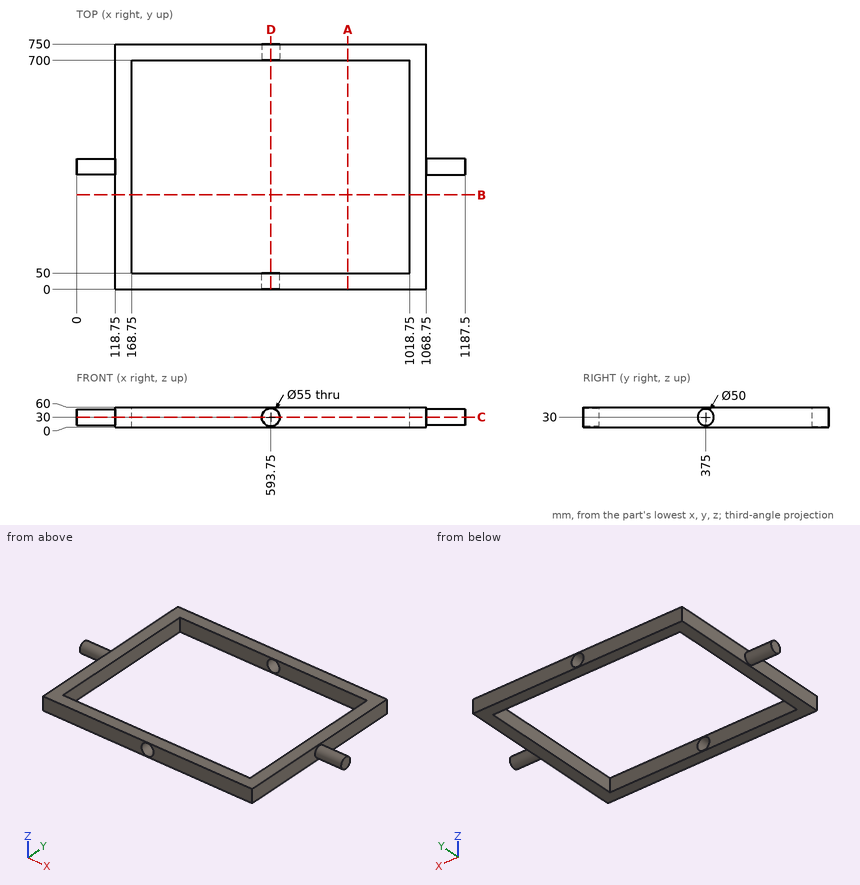
Could you check a few things on this drawing? It's one solid part, dimensions in mm from its lowest x, y, z. Give positions to 0.01 mm unless a question says otherwise; leave off trailing zeros. Order: outer loops, then holes, each group sorted by start corner. A loop starts at its lowest first (then second) coordinate and runs counter-clockwise, first axis right, second up.
1. Suppose I cut it at D-D (x = 593.75). Write out the boundary of the cut face in (y, z).
Answers below:
outline: (0, 0) - (50, 0) - (50, 2.5) - (0, 2.5) - close; (0, 57.5) - (50, 57.5) - (50, 60) - (0, 60) - close; (700, 0) - (750, 0) - (750, 2.5) - (700, 2.5) - close; (700, 57.5) - (750, 57.5) - (750, 60) - (700, 60) - close
2. Suppose I cut it at A-A (x = 829). Write out the boundary of the cut face in (y, z), plus the area to 3 significant figures.
Answers below:
outline: (0, 0) - (50, 0) - (50, 60) - (0, 60) - close; (700, 0) - (750, 0) - (750, 60) - (700, 60) - close
area: 6,000 mm2
3. For pin 1 (2 mm diameter, centred on x = 570.5, z = 39, fed in from -Y); pin 2 (4 mm diameter, centred on y = 651.5, z = 45.5, fed in from +X), each with a flat end and sliding along its axis, tell me the tip position at first contact or that it passes through.
Answers below:
pin 1: passes through
pin 2: stops at x = 1068.75
4. Suppose I cut it at C-C (z = 30). Write out the boundary of the cut face in (x, y), plus the area to 3 significant figures.
Answers below:
outline: (0, 350) - (118.75, 350) - (118.75, 0) - (566.25, 0) - (566.25, 50) - (168.75, 50) - (168.75, 700) - (566.25, 700) - (566.25, 750) - (118.75, 750) - (118.75, 400) - (0, 400) - close; (621.25, 0) - (1068.75, 0) - (1068.75, 350) - (1187.5, 350) - (1187.5, 400) - (1068.75, 400) - (1068.75, 750) - (621.25, 750) - (621.25, 700) - (1018.75, 700) - (1018.75, 50) - (621.25, 50) - close
area: 166,000 mm2
5. Suppose I cut it at B-B (y = 289). Write out the boundary of the cut face in (x, z).
Answers below:
outline: (118.75, 0) - (168.75, 0) - (168.75, 60) - (118.75, 60) - close; (1018.75, 0) - (1068.75, 0) - (1068.75, 60) - (1018.75, 60) - close
6. I need wall thicknesses on L1, parallel to X at y = 551.5, z = 17; L2, parallel to X at y = 382.5, z = 29.5; L3, parallel to Y at x = 395, z = 4. Which ranges of each line are inside material? Lowest first, please.
Answers below:
L1: x = 118.75 to 168.75, 1018.75 to 1068.75
L2: x = 0 to 168.75, 1018.75 to 1187.5
L3: y = 0 to 50, 700 to 750
